Part print with two shaded views. Sizes in mm from the minimum x, y, z corner. A direction names the side the tool comes from. Coordinates: 2 decimals unless noted, no trailing zeros. Order: outer loops, then holes, each group sorted by start corner. A loop starts at its lowest first (then second) coordinate and runs counter-clockwise, first axis right, second up.
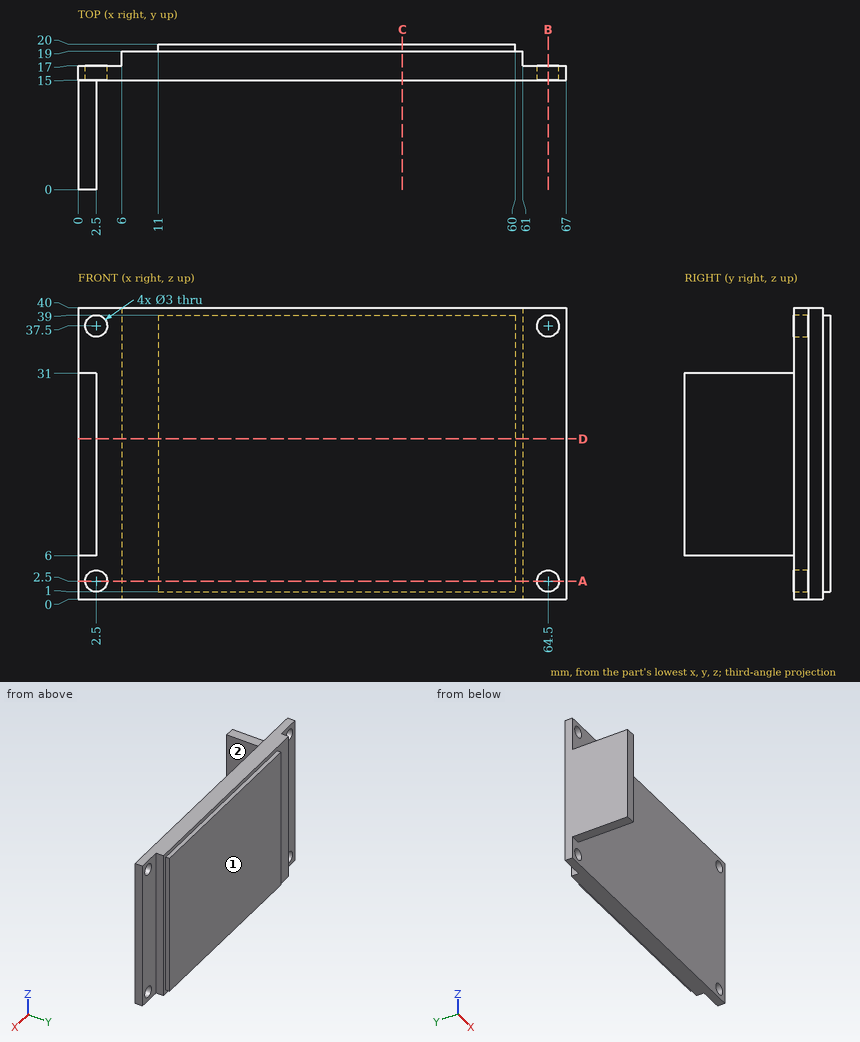
Q1. Cut at A-A on z = 2.5. Write the cut outline in (x, y).
Results list:
outline: (0, 15) - (1, 15) - (1, 17) - (0, 17) - close; (4, 15) - (63, 15) - (63, 17) - (61, 17) - (61, 19) - (60, 19) - (60, 20) - (11, 20) - (11, 19) - (6, 19) - (6, 17) - (4, 17) - close; (66, 15) - (67, 15) - (67, 17) - (66, 17) - close
Q2. Cut at C-C on x = 44.5. Write the cut outline in (y, z).
Results list:
outline: (15, 0) - (19, 0) - (19, 1) - (20, 1) - (20, 39) - (19, 39) - (19, 40) - (15, 40) - close
Q3. Cut at B-B on x = 64.5. Write the cut outline in (y, z), and give its area (3 significant figures).
Results list:
outline: (15, 0) - (17, 0) - (17, 1) - (15, 1) - close; (15, 4) - (17, 4) - (17, 36) - (15, 36) - close; (15, 39) - (17, 39) - (17, 40) - (15, 40) - close
area: 68.0 mm2
Q4. Which spindle directions (+Z, -Z, +X, -X, +Y, -Y) get a long thin tool onto all of the face, cutting with end or side? Do the marked faces 1 and 2. Say none if no direction does.
Results list:
face 1: +Z, -Z, +X, -X, +Y
face 2: +Z, -Z, +X, -Y
Q5. Pin check, flat tips, straight feed: pin 1 Ø0.8 at (x, y) = (1.5, 5.5) entering from -Z; pin 2 Ø1 at (y, z) = (18, 14) entering from -X; pin 3 Ø4 at (x, z) = (2.5, 2.5) entering from +Y; pin 4 Ø6.5 at (x, z) = (62.5, 11.5) entering from +Y. Stop position of each tip, or through.
Results list:
pin 1: stops at z = 6
pin 2: stops at x = 6
pin 3: stops at y = 17
pin 4: stops at y = 20
Q6. Cut at D-D on z = 22. Write the cut outline in (x, y), and give its area (4 significant figures).
Results list:
outline: (0, 0) - (2.5, 0) - (2.5, 15) - (67, 15) - (67, 17) - (61, 17) - (61, 19) - (60, 19) - (60, 20) - (11, 20) - (11, 19) - (6, 19) - (6, 17) - (0, 17) - close
area: 330.5 mm2
Q7. Wall check: line 1 along X through (y, z) = (16.3, 2.5); line 2 along Z through (x, y) = (64.5, 15.8); line 3 along X through (y, z) = (4.5, 24.5). Give the ranges that are in metal, low to high.
Results list:
line 1: x = 0 to 1, 4 to 63, 66 to 67
line 2: z = 0 to 1, 4 to 36, 39 to 40
line 3: x = 0 to 2.5
